```python
from build123d import *

# Parameters (mm, degrees)
EXTRUDE1_DEPTH            = 6
SKETCH2_W                 = 44
SKETCH2_H                 = 44
EXTRUDE2_DEPTH            = 3
SKETCH4_R                 = 32.5
EXTRUDE3_DEPTH            = 17.5
SKETCH3_R                 = 9.5
EXTRUDE4_DEPTH            = 27.5
SKETCH16_R                = 21
EXTRUDE7_DEPTH            = 12
SKETCH19_R                = 2.5
EXTRUDE8_DEPTH            = 24.5
LPATTERN1_COUNT           = 2
LPATTERN1_PITCH           = 56
LPATTERN2_COUNT           = 2
LPATTERN2_PITCH           = 56
LPATTERN2_COPY_1_SKETCH_R = 2.5
LPATTERN2_COPY_1_DEPTH    = 24.5


with BuildPart() as part:
    # Sketch1 → Extrude1 (new body)
    with BuildSketch(Plane(origin=(0, 0, 0), x_dir=(0, 0, -1), z_dir=(1, 0, 0))):
        Polygon((0, 68), (9, 77), (68, 77), (77, 68), (77, 9), (68, 0), (9, 0), (0, 9), align=None)
    extrude(amount=EXTRUDE1_DEPTH)

    # Sketch2 → Extrude2 (add)
    with BuildSketch(Plane(origin=(6, 0, 0), x_dir=(0, 0, -1), z_dir=(1, 0, 0))):
        with Locations((38.5, 38.5)):
            Rectangle(SKETCH2_W, SKETCH2_H)
    extrude(amount=EXTRUDE2_DEPTH)

    # Sketch4 → Extrude3 (add)
    with BuildSketch(Plane.ZY):
        with Locations((-38.5, 38.5)):
            Circle(SKETCH4_R)
    extrude(amount=EXTRUDE3_DEPTH)

    # Sketch3 → Extrude4 (cut, through all)
    with BuildSketch(Plane(origin=(9, 0, 0), x_dir=(0, 0, -1), z_dir=(1, 0, 0))):
        with Locations((38.5, 38.5)):
            Circle(SKETCH3_R)
    extrude(amount=-EXTRUDE4_DEPTH, mode=Mode.SUBTRACT)

    # Sketch16 → Extrude7 (cut)
    with BuildSketch(Plane.ZY.offset(17.5)):
        with Locations((-38.5, 38.5)):
            Circle(SKETCH16_R)
    extrude(amount=-EXTRUDE7_DEPTH, mode=Mode.SUBTRACT)

    # Sketch18 → Revolve2 (revolve)
    with BuildSketch(Plane.XZ.offset(-38.5)):
        Polygon((-5.5, -56.5), (-5.5, -59.5), (-17.5, -59.5), align=None)
    revolve(axis=Axis((9, 38.5, -38.5), (-1, 0, 0)))

    # Sketch19 → Extrude8 (cut, through all)
    with BuildSketch(Plane(origin=(6, 0, 0), x_dir=(0, 0, -1), z_dir=(1, 0, 0))):
        with Locations((10.5, 66.5)):
            Circle(SKETCH19_R)
    extrude8 = extrude(amount=-EXTRUDE8_DEPTH, mode=Mode.SUBTRACT)

    # LPattern1: Extrude8 ×2
    with Locations(*[(0, 0, -i * LPATTERN1_PITCH) for i in range(1, LPATTERN1_COUNT)]):
        add(extrude8, mode=Mode.SUBTRACT)

    # LPattern2: Extrude8 ×2
    with Locations(*[(0, -i * LPATTERN2_PITCH, 0) for i in range(1, LPATTERN2_COUNT)]):
        add(extrude8, mode=Mode.SUBTRACT)

    # LPattern2 copy 1 sketch → LPattern2 copy 1 (cut, through all)
    with BuildSketch(Plane(origin=(6, -56, -56), x_dir=(0, 0, -1), z_dir=(1, 0, 0))):
        with Locations((10.5, 66.5)):
            Circle(LPATTERN2_COPY_1_SKETCH_R)
    extrude(amount=-LPATTERN2_COPY_1_DEPTH, mode=Mode.SUBTRACT)


solid = part.part
```
Can you work these out from the model? Positions are in its coordinate system, mm. A direction names the side the tool comes from. Give positions to 0.01 mm unless a question says otherwise; leave off trailing zeros. Order: outer loops, then holes, each group sorted by start corner. A loop starts at its lowest first (then second) coordinate and runs counter-clockwise, first axis right, second up. Notation, with made-up numbers: (-9, -29) - (45, -29) arc R18 cw to (45, -1) - close; hole circle Ø5 at (69.25, 32.25). An arc over 180 degrees is marked (long way). Use a Markdown table: item, result. Add a question column.
Q1. If we section it at D-D on z = -10.5: Write out the boundary of the cut face in (x, y).
Q2. If we section it at C-C on x = 1.75: Write out the boundary of the cut face in (y, z).
Q3. If we section it at A-A on y = 10.5: Write out the boundary of the cut face in (x, z), plus the area to 4 significant figures.
Q4. I'm going to push flat-ended pins straight in: pin 1 (3.5 mm diameter, centred on x = 8, z = -35, fed in from +Y); pin 2 (2 mm diameter, centred on x = -13, z = -30.5, fed in from +Y); pin 3 (6 mm diameter, centred on y = 10.5, z = -10.5, fed in from -X). Where does each tip first touch, or does it pass through?
Q5. If we section it at B-B on z = -38.5: Write out the boundary of the cut face in (x, y).
Q6. If we mould it in two halves opening along Y, with no side actions, what happens to faces 1 (the flat face through (7, 16.5, -38)), 2 (the flat face through (-17.5, 39, -17)), 3 (the cylindrical face through (3.04, 64.28, -67.65))? For each: released by +Y, released by -Y, zero draft, split by the parting line, or undercut.
Q7. On a 3-axis mill with a long thin cutter (end or side, diameter ignored), from which of +Z, -Z, +X, -X, +Y, -Y can I reach the whole of each face in a straight line? I mean faces 4 (the flat face through (9, 49, -38)), 5 (the flat face through (7, 38, -16.5)), 6 (the cylindrical face through (-8.63, 39.93, -70.97)), 7 (the flat face through (7, 60.5, -38)). Say none if no direction works.
Q8. Please list where these lines run through material, in increasing order: line 1 along Y through (x, z) = (5.25, -66.5); line 2 along X through (y, z) = (13.5, -30.5); line 3 along Y through (x, z) = (-11.25, -54.5).
Answers follow:
| question | item | result |
|---|---|---|
| 1 | outline | (-17.5, 22) - (0, 22) - (0, 13) - (6, 13) - (6, 64) - (0, 64) - (0, 55) - (-17.5, 55) - close; (0, 0) - (6, 0) - (6, 8) - (0, 8) - close; (0, 69) - (6, 69) - (6, 77) - (0, 77) - close |
| 2 | outline | (0, -68) - (9, -77) - (68, -77) - (77, -68) - (77, -9) - (68, 0) - (9, 0) - (0, -9) - close; hole circle Ø5 at (10.5, -66.5); hole circle Ø5 at (10.5, -10.5); hole circle Ø19 at (38.5, -38.5); hole circle Ø5 at (66.5, -66.5); hole circle Ø5 at (66.5, -10.5) |
| 3 | outline | (-17.5, -55) - (0, -55) - (0, -64) - (6, -64) - (6, -13) - (0, -13) - (0, -22) - (-17.5, -22) - close; (0, -77) - (6, -77) - (6, -69) - (0, -69) - close; (0, -8) - (6, -8) - (6, 0) - (0, 0) - close |
| 3 | area | 979.5 mm^2 |
| 4 | pin 1 | stops at y = 60.5 |
| 4 | pin 2 | stops at y = 70.24 |
| 4 | pin 3 | stops at x = 0 |
| 5 | outline | (-17.5, 6) - (0, 6) - (0, 0) - (6, 0) - (6, 16.5) - (9, 16.5) - (9, 29) - (-5.5, 29) - (-5.5, 20.5) - (-17.5, 17.5) - close; (-17.5, 59.5) - (-5.5, 56.5) - (-5.5, 48) - (9, 48) - (9, 60.5) - (6, 60.5) - (6, 77) - (0, 77) - (0, 71) - (-17.5, 71) - close |
| 6 | face 1 | released by -Y |
| 6 | face 2 | zero draft |
| 6 | face 3 | undercut |
| 7 | face 4 | +Z, -Z, +X, +Y, -Y |
| 7 | face 5 | +Z, +X, +Y, -Y |
| 7 | face 6 | -X |
| 7 | face 7 | +Z, -Z, +X, +Y |
| 8 | line 1 | y = 0 to 8, 13 to 64, 69 to 77 |
| 8 | line 2 | x = -17.5 to 6 |
| 8 | line 3 | y = 10.21 to 27.46, 49.54 to 66.79 |
